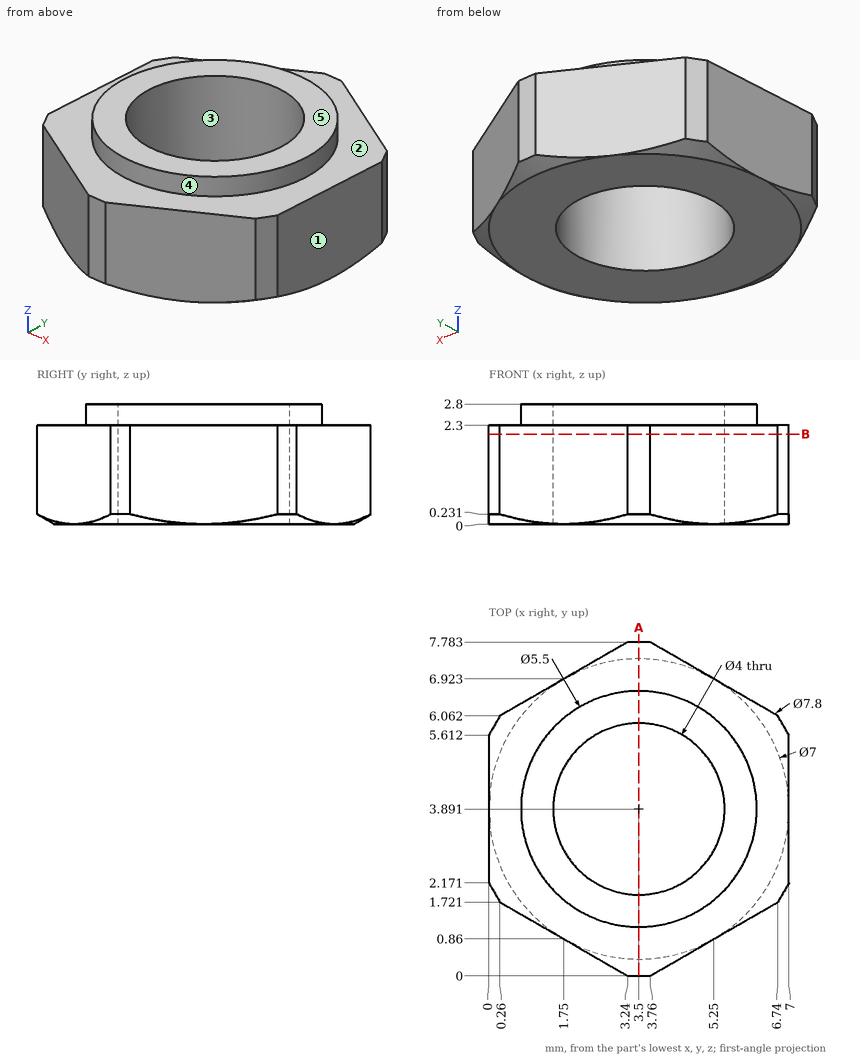
The drawing under review shows one solid part. Ordinate dimensions are in mm from its lowest x, y, z. A direction names the side the tool comes from. Coordinates: 2 decimals unless noted, no trailing zeros. Write each loop counter-clockwise with the first axis right and the second up, starting at its lowest first coordinate (ties: lowest second). Pieces come first, ordered by that corner, then holes.
1) Machinability: for the marked faces 1 and 2, which of the approach directions +Z, -Z, +X, -X, +Y, -Y give a long, thin tool a straight path to every point of the face, cutting with its end or side? Answer none if there is none.
2) Mouldability with a two-part tool opening along X and no side actions: class the marked faces 3, 4 and 5 as +X half, -X half, draft (parallel to the pull), parting line (faces both ways), or undercut.
3) To check wall thickness, follow L1, parallel to Y at x = 3.5, z = 2.05; L2, parallel to Z at x = 5.25, y = 1.25; L3, parallel to X at y = 4, z = 0.9. State the ranges of each line that lie inside material, in increasing order.
4) Insertion check: pin 1 (1 mm diameter, centred on x = 1, z = 2, fed in from -Y) (1 decimal). The pin has a flat end and moves straight along its axis. Give the tip position at first contact, or say it passes through.
5) Add section B-B (z = 2.1). Write out the cut boundary in (x, y).
6) Add section A-A (x = 3.5). Write out the cut boundary in (y, z).
Check result:
1. face 1: +Z, -Z, +X, +Y, -Y
1. face 2: +Z
2. face 3: undercut
2. face 4: parting line
2. face 5: draft
3. L1: y = 0 to 1.89, 5.89 to 7.78
3. L2: z = 0 to 2.3
3. L3: x = 0 to 1.5, 5.5 to 7
4. pin 1: stops at y = 1
5. outline: (0, 2.17) - (0.26, 1.72) - (3.24, 0) - (3.76, 0) - (6.74, 1.72) - (7, 2.17) - (7, 5.61) - (6.74, 6.06) - (3.76, 7.78) - (3.24, 7.78) - (0.26, 6.06) - (0, 5.61) - close; hole circle Ø4 at (3.5, 3.89)
6. outline: (0, 0.23) - (0.39, 0) - (1.89, 0) - (1.89, 2.8) - (1.14, 2.8) - (1.14, 2.3) - (0, 2.3) - close; (5.89, 0) - (7.39, 0) - (7.78, 0.23) - (7.78, 2.3) - (6.64, 2.3) - (6.64, 2.8) - (5.89, 2.8) - close
